from build123d import *

# Parameters (mm, degrees)
EXTRUDE_1_DEPTH   = 1
HOLE_WIZARD_M31_D = 3.4


with BuildPart() as part:
    # Эскиз1 → Бобышка-Вытянуть1 (new body)
    with BuildSketch(Plane(origin=(0, 0, 0), x_dir=(1, 0, 0), z_dir=(0, 1, 0))):
        with BuildLine():
            Line((22.325097984, -2.8), (25.3, -2.8))
            ThreePointArc((25.3, -2.8), (28.1, 0), (25.3, 2.8))
            Line((25.3, 2.8), (22.325097984, 2.8))
            ThreePointArc((22.325097984, 2.8), (15.909902577, 15.909902577), (2.8, 22.325097984))
            Line((2.8, 22.325097984), (2.8, 25.3))
            ThreePointArc((2.8, 25.3), (0, 28.1), (-2.8, 25.3))
            Line((-2.8, 25.3), (-2.8, 22.325097984))
            ThreePointArc((-2.8, 22.325097984), (-15.909902577, 15.909902577), (-22.325097984, 2.8))
            Line((-22.325097984, 2.8), (-25.3, 2.8))
            ThreePointArc((-25.3, 2.8), (-28.1, 0), (-25.3, -2.8))
            Line((-25.3, -2.8), (-22.325097984, -2.8))
            ThreePointArc((-22.325097984, -2.8), (-15.909902577, -15.909902577), (-2.8, -22.325097984))
            Line((-2.8, -22.325097984), (-2.8, -25.3))
            ThreePointArc((-2.8, -25.3), (0, -28.1), (2.8, -25.3))
            Line((2.8, -25.3), (2.8, -22.325097984))
            ThreePointArc((2.8, -22.325097984), (14.4243682, -14.4243682), (22.325097984, -2.8))
        make_face()
        with BuildLine():
            ThreePointArc((20.373939602, -2.269930633), (-14.495689014, 14.495689014), (2.269930633, -20.373939602))
            ThreePointArc((2.269930633, -20.373939602), (13.010154638, -13.010154638), (20.373939602, -2.269930633))
        make_face(mode=Mode.SUBTRACT)
    extrude(amount=EXTRUDE_1_DEPTH)

    # Отверстие с зазором M31 (through all)
    with Locations(Plane(origin=(0, 1, 0), x_dir=(1, 0, 0), z_dir=(0, 1, 0))):
        with Locations((-25.3, 0), (0, 25.3), (25.3, 0), (0, -25.3)):
            Hole(HOLE_WIZARD_M31_D / 2)


solid = part.part
Read the model definition and answer for the solid it produces. Units are mm, in the model's axes. A direction names the side the tool comes from. Give positions to 0.01 mm unless a question says otherwise; leave off trailing zeros. Write each loop counter-clockwise with the first axis right and the second up, starting at its lowest first coordinate (ties: lowest second). Pieces come first, ordered by that corner, then holes. Notation, with made-up numbers: (-39, 27.5) -> (12, 27.5) arc R14 cw to (12, 52.5) -> close; hole circle Ø10 at (80, 53.25). An arc over 180 degrees is marked (long way). Answer as a JSON object with one key per item and string values. Group by question number.
1) Find section A-A (y = 0.35). Write down the section's boundary in (x, z).
2) Find section B-B (x = 0). Write down the section's boundary in (y, z).
3) Consider L1, parallel to Z at x = 0, y = 0.35; L2, parallel to X at y = 0.4, z = -25.3. Determine where each line is inside the solid, lowest interval first. Write a range as from..to.
4) Find section D-D (x = -8). Write down the section's boundary in (y, z).
5) The mould has two halves that part along Z. Classify faces 1 (the cylindrical face through (0.1, 0.5, -28.1)), 2 (the cylindrical face through (-23.6, 0.49, -0.07)), 3 (the flat face through (12.4, 1, 14.4)): +Z half, -Z half, draft (parallel to the pull), parting line (faces both ways), or undercut.
6) Each of these flat-tipped pins is pushed along its axis until it touches: P1, Ø4, axis at x = 0, z = -25.3, coming from the +Y side; P2, Ø2, axis at x = 25.3, z = 0, coming from the +Y side. Where does it stop, or does it pass through?
7) Find section C-C (z = -19). Write down the section's boundary in (x, y).
8) A tool of negligible diameter and unlimited length cuts with its end or side. For faces 4 (the flat face through (12.4, 0, 14.4)), 5 (the cylindrical face through (12.88, 0.49, 13.14)), from which of +Z, -Z, +X, -X, +Y, -Y can it reach the whole face along a straight path? Write none if from no direction.
Values follow:
{
 "1": {"outline": "(-25.3, -2.8) -> (-22.33, -2.8) arc R22.5 ccw to (-2.8, -22.33) -> (-2.8, -25.3) arc R2.8 ccw to (2.8, -25.3) -> (2.8, -22.33) arc R22.5 ccw to (22.33, -2.8) -> (25.3, -2.8) arc R2.8 ccw to (25.3, 2.8) -> (22.33, 2.8) arc R37.51 ccw to (2.8, 22.33) -> (2.8, 25.3) arc R2.8 ccw to (-2.8, 25.3) -> (-2.8, 22.33) arc R22.5 ccw to (-22.33, 2.8) -> (-25.3, 2.8) arc R2.8 ccw to start; hole circle Ø3.4 at (-25.3, 0); hole circle Ø3.4 at (0, -25.3); hole circle Ø3.4 at (0, 25.3); hole (2.27, 20.37) arc R20.5 ccw (long way) to (20.37, 2.27) arc R35.51 ccw to start; hole circle Ø3.4 at (25.3, 0)"},
 "2": {"outline": "(0, -28.1) -> (1, -28.1) -> (1, -27) -> (0, -27) -> close; (0, -23.6) -> (1, -23.6) -> (1, -20.5) -> (0, -20.5) -> close; (0, 20.5) -> (1, 20.5) -> (1, 23.6) -> (0, 23.6) -> close; (0, 27) -> (1, 27) -> (1, 28.1) -> (0, 28.1) -> close"},
 "3": {"L1": "z = -28.1..-27, -23.6..-20.5, 20.5..23.6, 27..28.1", "L2": "x = -2.8..-1.7, 1.7..2.8"},
 "4": {"outline": "(0, -21.03) -> (1, -21.03) -> (1, -18.87) -> (0, -18.87) -> close; (0, 18.87) -> (1, 18.87) -> (1, 21.03) -> (0, 21.03) -> close"},
 "5": {"face 1": "-Z half", "face 2": "undercut", "face 3": "draft"},
 "6": {"P1": "stops at y = 1", "P2": "passes through"},
 "7": {"outline": "(-12.05, 0) -> (-7.7, 0) -> (-7.7, 1) -> (-12.05, 1) -> close; (7.7, 0) -> (12.05, 0) -> (12.05, 1) -> (7.7, 1) -> close"},
 "8": {"face 4": "+Z, -Z, +X, -X, -Y", "face 5": "+Y, -Y"}
}
